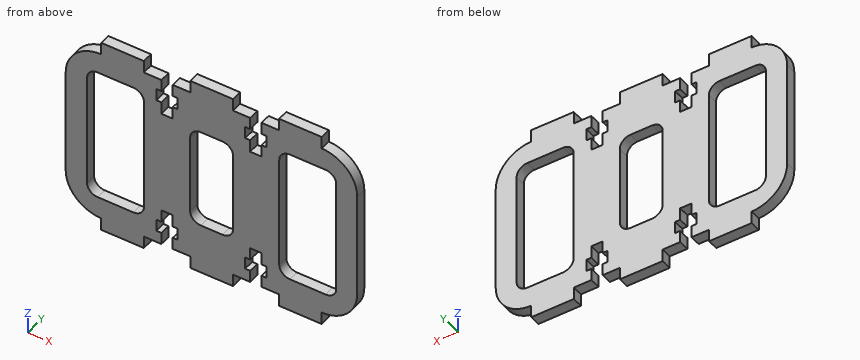
```python
from build123d import *

# Parameters (mm, degrees)
EXTRUDE_1_DEPTH     = 3
FILLET_1_R          = 10
SKETCH_2_W          = 12.1
SKETCH_2_H          = 28.4
SKETCH_2_W_2        = 16.05
SKETCH_2_H_2        = 38
CUT_EXTRUDE_1_DEPTH = 99.039073843
FILLET_2_R          = 3


with BuildPart() as part:
    # 草图1 → 凸台-拉伸1 (new body)
    with BuildSketch(Plane(origin=(0, 0, 0), x_dir=(1, 0, 0), z_dir=(0, 1, 0))):
        Polygon((10, 0), (10, -3.5), (22, -3.5), (22, 0), (26.95, 0), (26.95, 3.4), (25.55, 3.4), (25.55, 6.8), (26.95, 6.8), (26.95, 10.3), (30.15, 10.3), (30.15, 6.8), (31.55, 6.8), (31.55, 3.4), (30.15, 3.4), (30.15, 0), (35.1, 0), (35.1, -3.5), (47.1, -3.5), (47.1, 0), (51.95, 0), (51.95, 3.4), (50.55, 3.4), (50.55, 6.8), (51.95, 6.8), (51.95, 10.3), (55.15, 10.3), (55.15, 6.8), (56.55, 6.8), (56.55, 3.4), (55.15, 3.4), (55.15, 0), (60.1, 0), (60.1, -3.5), (72.1, -3.5), (72.1, 0), (82.1, 0), (82.1, 50), (72.1, 50), (72.1, 53.5), (60.1, 53.5), (60.1, 50), (55.15, 50), (55.15, 46.6), (56.55, 46.6), (56.55, 43.2), (55.15, 43.2), (55.15, 39.7), (51.95, 39.7), (51.95, 43.2), (50.55, 43.2), (50.55, 46.6), (51.95, 46.6), (51.95, 50), (47.1, 50), (47.1, 53.5), (35.1, 53.5), (35.1, 50), (30.15, 50), (30.15, 46.6), (31.55, 46.6), (31.55, 43.2), (30.15, 43.2), (30.15, 39.7), (26.95, 39.7), (26.95, 43.2), (25.55, 43.2), (25.55, 46.6), (26.95, 46.6), (26.95, 50), (22, 50), (22, 53.5), (10, 53.5), (10, 50), (0, 50), (0, 0), align=None)
    extrude(amount=EXTRUDE_1_DEPTH)

    # 圆角1
    fillet_1_edges = [part.edges().sort_by_distance(p)[0] for p in [
        (0, 1.5, -50),
        (82.1, 1.5, -50),
        (82.1, 1.5, 0),
        (0, 1.5, 0),
    ]]
    fillet(fillet_1_edges, radius=FILLET_1_R - 0.0001)  # a hair under: the kernel refuses the full size

    # 草图2 → 切除-拉伸1 (cut, through all)
    with BuildSketch(Plane.XZ):
        with Locations((41.1, -25)):
            Rectangle(SKETCH_2_W, SKETCH_2_H)
        with Locations((14.025, -25)):
            Rectangle(SKETCH_2_W_2, SKETCH_2_H_2)
        with Locations((68.175, -25)):
            Rectangle(SKETCH_2_W_2, SKETCH_2_H_2)
    extrude(amount=-CUT_EXTRUDE_1_DEPTH, mode=Mode.SUBTRACT)

    # 圆角2
    fillet_2_edges = [part.edges().sort_by_distance(p)[0] for p in [
        (60.15, 1.5, -6),
        (76.2, 1.5, -6),
        (76.2, 1.5, -44),
        (60.15, 1.5, -44),
        (6, 1.5, -44),
        (6, 1.5, -6),
        (22.05, 1.5, -6),
        (22.05, 1.5, -44),
        (35.05, 1.5, -39.2),
        (35.05, 1.5, -10.8),
        (47.15, 1.5, -10.8),
        (47.15, 1.5, -39.2),
    ]]
    fillet(fillet_2_edges, radius=FILLET_2_R)


solid = part.part
```
Source: CAD feature listing. Evaluate the final solid. Frame: model axes, mm. Give positions to 0.01 mm unless a question says otherwise; leave off trailing zeros. Order: outer loops, then holes, each group sorted by start corner. A loop starts at its lowest first (then second) coordinate and runs counter-clockwise, first axis right, second up. Notation, with made-up numbers: (14.25, 69) -> (60.25, 69) arc R21 cw to (60.25, 96) -> close; hole circle Ø6 at (13, 69). An arc over 180 degrees is marked (long way). Use a Markdown table: item, result.
Q1. First-contact query: P1, Ø1.5, axis at y = 2, z = -46.5, coming from the +X side; P2, Ø1.1, axis at x = 30.5, y = 1, coming from the -Z side; P3, Ø0.9, axis at y = 2, z = -51.5, coming from the -X side. Flat tips, straight axial feed; report the tip coordinate or a pass-through.
A:
| item | result |
|---|---|
| P1 | x = 80.28 |
| P2 | z = -50 |
| P3 | x = 10 |
Q2. Material intervals for line 1 (X direction, y = 0.2, z = -17); line 2 (Z direction, x = 26, y = 0.7); line 3 (X direction, y = 2.2, z = -39.5), sorted ascending. Write a range as [from, to].
A:
| item | result |
|---|---|
| line 1 | [0, 6], [22.05, 35.05], [47.15, 60.15], [76.2, 82.1] |
| line 2 | [-50, -46.6], [-43.2, -6.8], [-3.4, 0] |
| line 3 | [0, 6], [22.05, 60.15], [76.2, 82.1] |
Q3. Section B-B (z = -5). Return the cut outline in (x, y).
A:
| item | result |
|---|---|
| outline | (1.34, 0) -> (25.55, 0) -> (25.55, 3) -> (1.34, 3) -> close; (31.55, 0) -> (50.55, 0) -> (50.55, 3) -> (31.55, 3) -> close; (56.55, 0) -> (80.76, 0) -> (80.76, 3) -> (56.55, 3) -> close |
Q4. Section C-C (z = -26). Return the cut outline in (x, y).
A:
| item | result |
|---|---|
| outline | (0, 0) -> (6, 0) -> (6, 3) -> (0, 3) -> close; (22.05, 0) -> (35.05, 0) -> (35.05, 3) -> (22.05, 3) -> close; (47.15, 0) -> (60.15, 0) -> (60.15, 3) -> (47.15, 3) -> close; (76.2, 0) -> (82.1, 0) -> (82.1, 3) -> (76.2, 3) -> close |
Q5. Section D-D (x = 40). Return the cut outline in (y, z), and give its area (3 significant figures).
A:
| item | result |
|---|---|
| outline | (0, -53.5) -> (3, -53.5) -> (3, -39.2) -> (0, -39.2) -> close; (0, -10.8) -> (3, -10.8) -> (3, 3.5) -> (0, 3.5) -> close |
| area | 85.8 mm^2 |
Q6. Section A-A (x = 69). Return the cut outline in (y, z).
A:
| item | result |
|---|---|
| outline | (0, -53.5) -> (3, -53.5) -> (3, -44) -> (0, -44) -> close; (0, -6) -> (3, -6) -> (3, 3.5) -> (0, 3.5) -> close |
